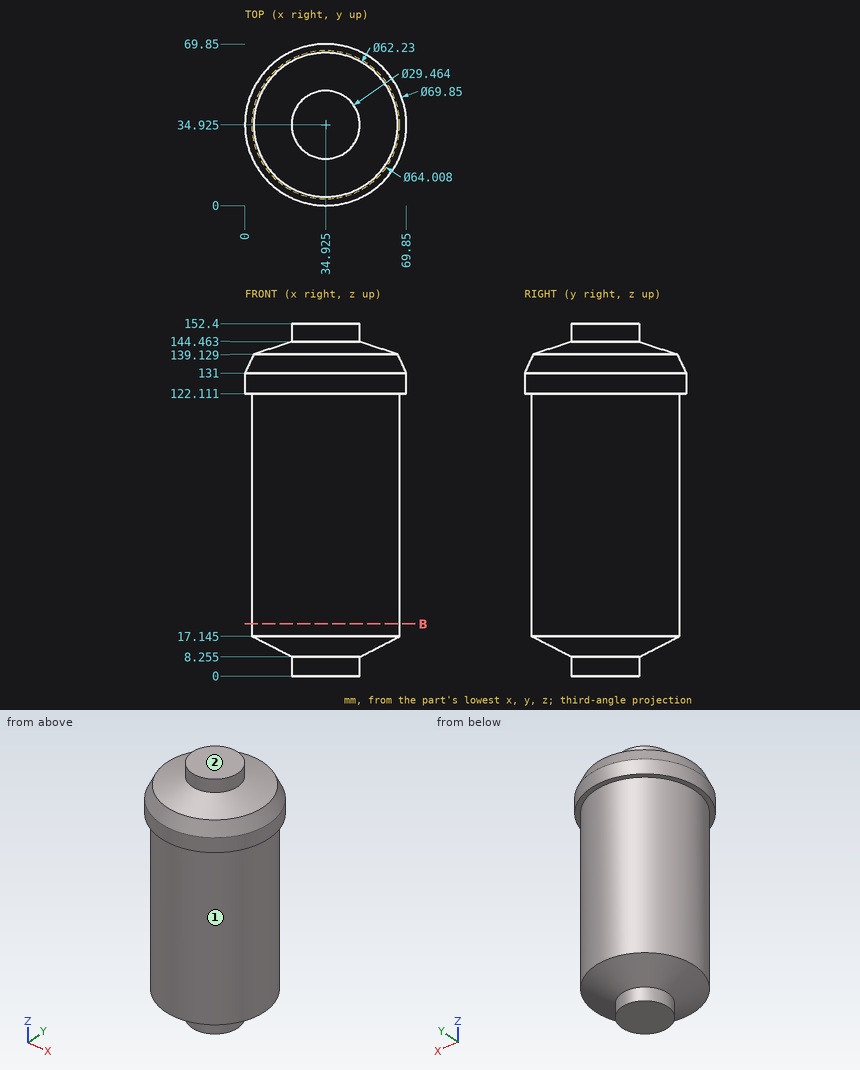
Drawing for the job (mm, zero at the part's lowest x, y, z). A direction names the side the tool comes from. Coordinates: 2 decimals unless noted, no trailing zeros. Order: outer loops, then holes, each group sorted by start corner. A loop starts at its lowest first (then second) coordinate and runs counter-clockwise, first axis right, second up. Notation, with made-up numbers: (43.25, 2.5) - (49.25, 2.5) arc R16 ccw to (49.25, 9.5) - close; hole circle Ø10 at (34.25, -20.75). An arc over 180 degrees is marked (long way). Use a Markdown table: item, result. Add a question column.
(1) Saw through at B-B (z = 22.5). Give the cut face in (x, y) (1 decimal).
(2) Flat gauge pins, fed straight in: pin 1 (4 mm diameter, centred on x = 14.5, z = 37, fed in from -Y); pin 2 (12 mm diameter, centred on x = 49, z = 76, fed in from +Y); pin 3 (12 mm diameter, centred on y = 51.5, z = 136, fed in from -X). Where does each tip first touch, or does it go through?
(3) Drill centre lines: line 1 along Y through (x, z) = (31, 131); line 2 along Z through (x, y) = (22.5, 54.5) (1 decimal); line 3 along X through (y, z) = (26, 71.5). Where is each one in solid material? Low to high. Write a range as [from, to].
(4) Which spindle directions (+Z, -Z, +X, -X, +Y, -Y) get a long thin tool onto all of the face, cutting with end or side? Do the marked faces 1 and 2. Say none if no direction does.
Solved:
| question | item | result |
|---|---|---|
| 1 | outline | circle Ø64 at (34.9, 34.9) |
| 2 | pin 1 | stops at y = 8.76 |
| 2 | pin 2 | stops at y = 65.89 |
| 2 | pin 3 | stops at x = 2.6 |
| 3 | line 1 | y = [0.22, 69.63] |
| 3 | line 2 | z = [12.6, 141.7] |
| 3 | line 3 | x = [4.19, 65.66] |
| 4 | face 1 | -Z |
| 4 | face 2 | +Z, +X, -X, +Y, -Y |
